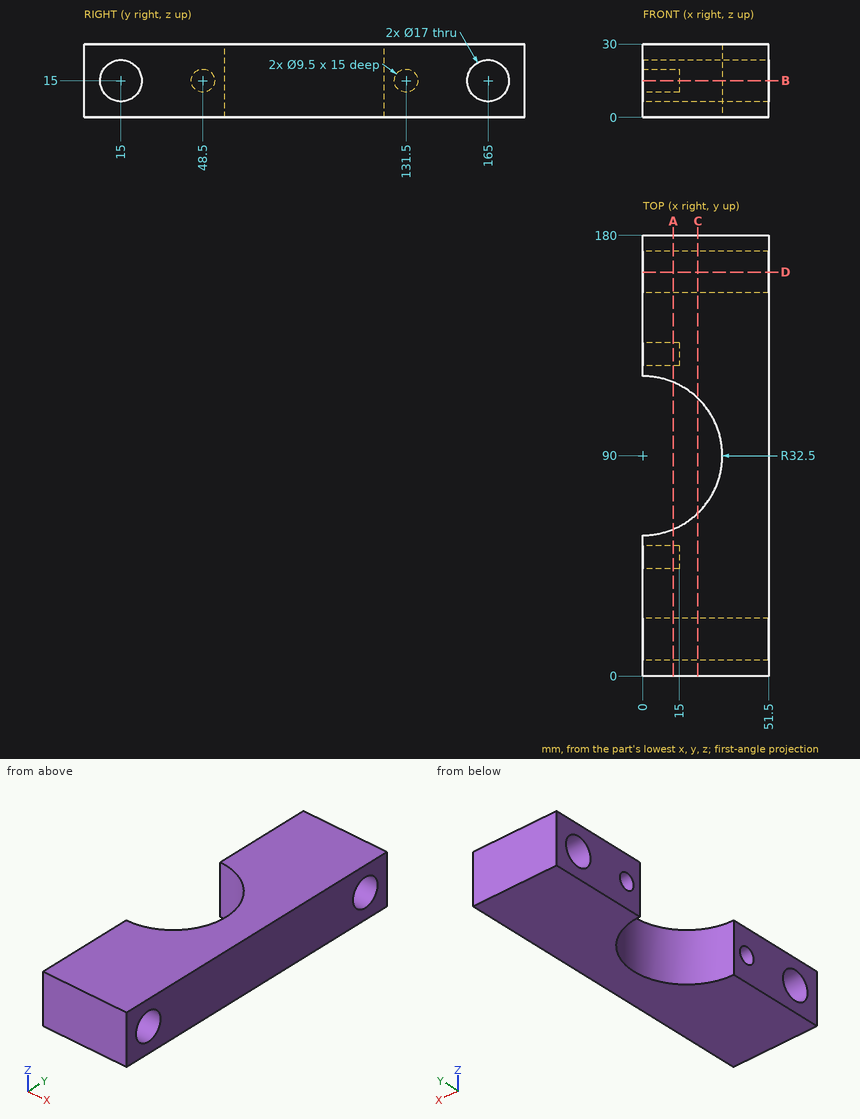
Geometry: see drawing. Coordinates: mm, zero at the bounding-box minimum. Round coordinates to 2 decimals unless told otherwise and drop trailing zeros. Write each loop counter-clockwise with the first axis right and the second up, starting at its lowest first coordinate (ties: lowest second). Pieces come first, ordered by that corner, then holes.
Item 1: Pin query (flat end, axial travel): P1, Ø7.5, axis at y = 48.5, z = 15, coming from the -X side. Return the tip coordinate at first contact, or that it passes through.
Item 2: Section query A-A (x = 12.5). Return loops of the section in (y, z).
Item 3: Section query D-D (y = 165). Return loops of the section in (x, z).
Item 4: Material intervals for L1, parallel to Y at x = 39.5, z = 15; L2, parallel to Y at x = 45.5, z = 14; L3, parallel to Y at x = 25, z = 14.25, sorted ascending.
Item 5: Section query C-C (x = 22.5). Return loops of the section in (y, z).
Item 6: Section query B-B (z = 15). Return loops of the section in (x, y), plus the area to 3 significant figures.
Completed:
1. P1: stops at x = 15
2. outline: (0, 0) - (60, 0) - (60, 30) - (0, 30) - close; (120, 0) - (180, 0) - (180, 30) - (120, 30) - close; hole circle Ø17 at (15, 15); hole circle Ø9.5 at (48.5, 15); hole circle Ø9.5 at (131.5, 15); hole circle Ø17 at (165, 15)
3. outline: (0, 0) - (51.5, 0) - (51.5, 6.5) - (0, 6.5) - close; (0, 23.5) - (51.5, 23.5) - (51.5, 30) - (0, 30) - close
4. L1: y = 0 to 6.5, 23.5 to 156.5, 173.5 to 180
4. L2: y = 0 to 6.56, 23.44 to 156.56, 173.44 to 180
4. L3: y = 0 to 6.53, 23.47 to 69.23, 110.77 to 156.53, 173.47 to 180
5. outline: (0, 0) - (66.55, 0) - (66.55, 30) - (0, 30) - close; (113.45, 0) - (180, 0) - (180, 30) - (113.45, 30) - close; hole circle Ø17 at (15, 15); hole circle Ø17 at (165, 15)
6. outline: (0, 0) - (51.5, 0) - (51.5, 6.5) - (0, 6.5) - close; (0, 23.5) - (51.5, 23.5) - (51.5, 156.5) - (0, 156.5) - (0, 136.25) - (15, 136.25) - (15, 126.75) - (0, 126.75) - (0, 122.5) arc R32.5 cw to (0, 57.5) - (0, 53.25) - (15, 53.25) - (15, 43.75) - (0, 43.75) - close; (0, 173.5) - (51.5, 173.5) - (51.5, 180) - (0, 180) - close
6. area: 5,570 mm2
